```python
from build123d import *

# Parameters (mm, degrees)
SKETCH_2_W               = 20
SKETCH_2_H               = 20
EXTRUDE_1_DEPTH          = 10
SKETCH_3_OUTSIDE_W       = 28.928
SKETCH_3_OUTSIDE_H       = 28.928
SKETCH_3_OUTSIDE_R       = 5
CUT_EXTRUDE_1_DEPTH      = 20
SKETCH_4_OUTSIDE_W       = 16.898
SKETCH_4_OUTSIDE_H       = 26.898
SKETCH_4_OUTSIDE_R       = 5
CUT_EXTRUDE_2_DEPTH      = 10
SKETCH_5_OUTSIDE_W       = 15.464
SKETCH_5_OUTSIDE_H       = 15.464
SKETCH_5_OUTSIDE_R       = 5
CUT_EXTRUDE_3_DEPTH      = 10
CUT_EXTRUDE_4_REACH      = 10.66
SKETCH_6_R               = 0.5
PATTERN_CIRCULAR_1_COUNT = 4
CUT_EXTRUDE_5_DEPTH      = 9.645808409
CUT_EXTRUDE_5_DEPTH_BACK = 9.645808409
SKETCH_7_R               = 0.5


with BuildPart() as part:
    # 草图2 → 凸台-拉伸1 (new, symmetric)
    with BuildSketch(Plane(origin=(0, 0, 0), x_dir=(1, 0, 0), z_dir=(0, 1, 0))):
        Rectangle(SKETCH_2_W, SKETCH_2_H)
    extrude(amount=EXTRUDE_1_DEPTH, both=True)

    # 草图3 outside → 切除-拉伸1 (cut)
    with BuildSketch(Plane.XY.offset(10)):
        Rectangle(SKETCH_3_OUTSIDE_W, SKETCH_3_OUTSIDE_H)
        Circle(SKETCH_3_OUTSIDE_R, mode=Mode.SUBTRACT)
    extrude(amount=-CUT_EXTRUDE_1_DEPTH, mode=Mode.SUBTRACT)

    # 草图4 outside → 切除-拉伸2 (cut, symmetric)
    with BuildSketch(Plane(origin=(0, 0, 0), x_dir=(1, 0, 0), z_dir=(0, 1, 0))):
        Rectangle(SKETCH_4_OUTSIDE_W, SKETCH_4_OUTSIDE_H)
        Circle(SKETCH_4_OUTSIDE_R, mode=Mode.SUBTRACT)
    extrude(amount=CUT_EXTRUDE_2_DEPTH, both=True, mode=Mode.SUBTRACT)

    # 草图5 outside → 切除-拉伸3 (cut, symmetric)
    with BuildSketch(Plane(origin=(0, 0, 0), x_dir=(0, 0, -1), z_dir=(1, 0, 0))):
        Rectangle(SKETCH_5_OUTSIDE_W, SKETCH_5_OUTSIDE_H)
        Circle(SKETCH_5_OUTSIDE_R, mode=Mode.SUBTRACT)
    extrude(amount=CUT_EXTRUDE_3_DEPTH, both=True, mode=Mode.SUBTRACT)

    # 草图6 → 切除-拉伸4 (cut, up to next)
    with BuildSketch(Plane(origin=(0, 0, 0), x_dir=(0, 0, -1), z_dir=(1, 0, 0)), mode=Mode.PRIVATE) as cut_extrude_4_sk1:
        Circle(SKETCH_6_R)
    cut_extrude_4_tool1 = extrude(cut_extrude_4_sk1.sketch, amount=-CUT_EXTRUDE_4_REACH, mode=Mode.PRIVATE) & part.part
    cut_extrude_4 = cut_extrude_4_tool1.solids().sort_by_distance((0, 0, 0))[0]
    add(cut_extrude_4, mode=Mode.SUBTRACT)

    # 阵列(圆周)1: 切除-拉伸4 ×4 about axis
    pattern_circular_1_axis = Axis((0, 5.5, 0), (0, -1, 0))
    for i in range(1, PATTERN_CIRCULAR_1_COUNT):
        add(cut_extrude_4.rotate(pattern_circular_1_axis, i * 360 / PATTERN_CIRCULAR_1_COUNT), mode=Mode.SUBTRACT)

    # 草图7 → 切除-拉伸5 (cut, two sides: drawn at the far end of the back side and taken through both)
    with BuildSketch(Plane(origin=(0, 0, 0), x_dir=(1, 0, 0), z_dir=(0, 1, 0)).offset(-CUT_EXTRUDE_5_DEPTH_BACK)):
        with Locations(Location((0, 0, 0), (0, 0, 314.999999812))):
            Circle(SKETCH_7_R)
    extrude(amount=CUT_EXTRUDE_5_DEPTH + CUT_EXTRUDE_5_DEPTH_BACK, mode=Mode.SUBTRACT)


solid = part.part
```
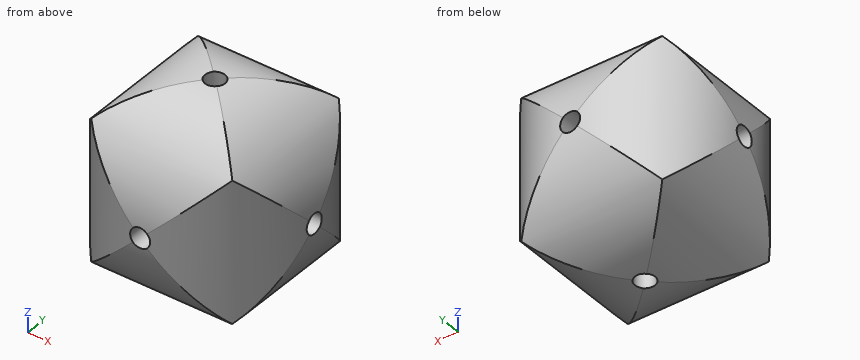
Here's how the part is built. I have some questions about the finished solid (model axes, mm). Coordinates: 2 decimals unless noted, no trailing zeros. Write each loop counter-clockwise with the first axis right and the second up, starting at its lowest first coordinate (ties: lowest second). Pieces come first, ordered by that corner, then holes. Notation, with made-up numbers: (52.5, -28.75) -> (110.5, -28.75) arc R12 cw to (110.5, -24.75) -> close; hole circle Ø4 at (25.25, 68). An arc over 180 degrees is marked (long way). Use a Markdown table: item, result. Add a question column.
(1) If we section it at C-C, the plane x = -4: Write out the boundary of the cut face in (y, z).
(2) I'm going to push flat-ended pins straight in: P1, Ø3, axis at y = 4, z = -1.5, coming from the -X side; P2, Ø3, axis at y = 3.5, z = 0, coming from the +X side; P3, Ø2, axis at y = -2, z = 2, coming from the -X side. Where does each tip first touch, or does it pass through?
(3) If we section it at A-A, the plane y = 0: Write out the boundary of the cut face in (x, z), and give its area (3 significant figures).
(4) Please list where these lines run through material, in increasing order: line 1 (Z direction, x = 0, y = -3.15); line 2 (Y direction, x = -2.5, z = 0); line 3 (X direction, y = -0.25, z = -2.75).
(5) If we section it at D-D, the plane y = 3.75: Write out the boundary of the cut face in (x, z), and give its area (3 significant figures).
Outcome:
| question | item | result |
|---|---|---|
| 1 | outline | (-3, -3) -> (3, -3) -> (3, 3) -> (-3, 3) -> close; hole circle Ø1 at (0, 0) |
| 2 | P1 | stops at x = -4.33 |
| 2 | P2 | stops at x = 4.58 |
| 2 | P3 | stops at x = -4.83 |
| 3 | outline | (-4.97, -0.5) arc R5 ccw to (-0.5, -4.97) -> (-0.5, -0.5) -> close; (-4.97, 0.5) -> (-0.5, 0.5) -> (-0.5, 4.97) arc R5 ccw to start; (0.5, -4.97) arc R5 ccw to (4.97, -0.5) -> (0.5, -0.5) -> close; (0.5, 0.5) -> (4.97, 0.5) arc R5 ccw to (0.5, 4.97) -> close |
| 3 | area | 59.6 mm^2 |
| 4 | line 1 | z = -3.88 to -0.5, 0.5 to 3.88 |
| 4 | line 2 | y = -4.33 to -0.5, 0.5 to 4.33 |
| 4 | line 3 | x = -4.18 to -0.43, 0.43 to 4.18 |
| 5 | outline | (-3.31, -3.31) -> (3.31, -3.31) -> (3.31, 3.31) -> (-3.31, 3.31) -> close; hole circle Ø1 at (0, 0) |
| 5 | area | 43.0 mm^2 |
